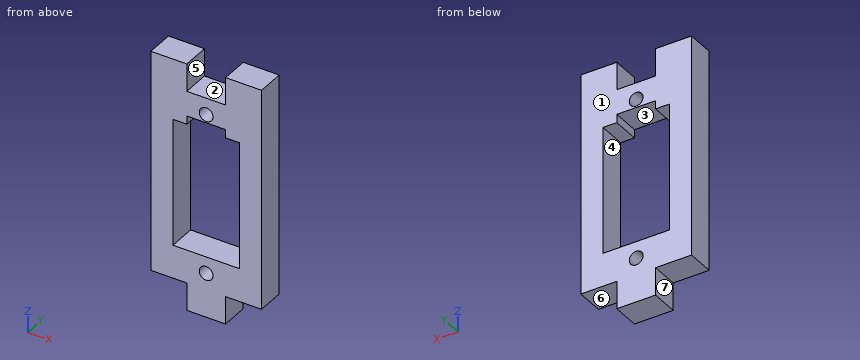
from build123d import *

# Parameters (mm, degrees)
BOSS_EXTRUDE1_DEPTH = 5
SKETCH2_R           = 1.25
CUT_EXTRUDE1_DEPTH  = 5


with BuildPart() as part:
    # Sketch1 → Boss-Extrude1 (new body)
    with BuildSketch(Plane(origin=(0, 0, 0), x_dir=(1, 0, 0), z_dir=(0, 1, 0))):
        Polygon((-10, 20), (-10, -20), (-3.5, -20), (-3.5, -15), (3.5, -15), (3.5, -20), (10, -20), (10, 20), (3.5, 20), (3.5, 25), (-3.5, 25), (-3.5, 20), align=None)
    extrude(amount=BOSS_EXTRUDE1_DEPTH)

    # Sketch2 → Cut-Extrude1 (cut)
    with BuildSketch(Plane(origin=(0, 5, 0), x_dir=(1, 0, 0), z_dir=(0, 1, 0))):
        with Locations(Location((0, 17, 0), (0, 0, 270))):
            Circle(SKETCH2_R)
        with Locations(Location((0, -12, 0), (0, 0, 270))):
            Circle(SKETCH2_R)
        Polygon((-6, 14), (6, 14), (6, -9), (3.5, -9), (3.5, -10.5), (-3.5, -10.5), (-3.5, -9), (-6, -9), align=None)
    extrude(amount=-CUT_EXTRUDE1_DEPTH, mode=Mode.SUBTRACT)


solid = part.part
The listing builds one solid part. Answer for the finished solid, in the listing's coordinates (mm). Face numbers are marked on the shaded views. A direction names the side the tool comes from. Round coordinates to 2 decimals unless told otherwise and drop trailing zeros. Write each loop counter-clockwise with the first axis right and the second up, starting at its lowest first coordinate (ties: lowest second). Pieces come first, ordered by that corner, then holes. Notation, with made-up numbers: (58, 38) - (69, 38) arc R30 ccw to (69, 76) - close; hole circle Ø9 at (-39, -17.75). An arc over 180 degrees is marked (long way). Use one line per item in the form item = value. Start each with the question number.
Item 1: A tool of negligible diameter and unlimited length cuts with its end or side. For the marked faces 4, 5, 6 and 7, from which of +Z, -Z, +X, -X, +Y, -Y can it reach the whole face along a straight path? Write none if from no direction.
Item 2: Find the intervals of material crossed by line 1 (Z direction, x = 2.25, y = 3.1); line 2 (X direction, y = 0.35, z = -9); line 3 (Z direction, x = 4.75, y = 0.55), in increasing order. Write a range as [from, to].
Item 3: A cutting plane is placed at D-D (x = 4.75). Write down the section's boundary in (y, z).
Item 4: A cutting plane is placed at A-A (x = 0). Write down the section's boundary in (y, z).
Item 5: Flat-ended cylindrical pins translate along their axes: pin 1 Ø1.5 at (x, y) = (-7, 2) entering from -Z; pin 2 Ø2.5 at (y, z) = (2.5, -22) entering from +X. Find the tip coordinate at first contact, or state that the pin passes through.
Item 6: Determine the mould class of the marked faces 1, 2 and 3 for opening direction Z: +Z half, -Z half, draft (parallel to the pull), parting line (faces both ways), or undercut.
Item 7: A cutting plane is placed at B-B (z = -17). Write down the section's boundary in (x, y), plus the area to 3 significant figures.
Item 8: A cutting plane is placed at C-C (y = 1.1). Write down the section's boundary in (x, z), plus the area to 3 significant figures.
The answers:
q1.face_4 = +Y, -Y
q1.face_5 = +Z, +Y, -Y
q1.face_6 = -Z, +X, +Y, -Y
q1.face_7 = -Z, -X, +Y, -Y
q2.line_1 = [-25, -14], [10.5, 15]
q2.line_2 = [-10, -6], [6, 10]
q2.line_3 = [-20, -14], [9, 20]
q3.outline = (0, -20) - (5, -20) - (5, -14) - (0, -14) - close; (0, 9) - (5, 9) - (5, 20) - (0, 20) - close
q4.outline = (0, -25) - (5, -25) - (5, -18.25) - (0, -18.25) - close; (0, -15.75) - (5, -15.75) - (5, -14) - (0, -14) - close; (0, 10.5) - (5, 10.5) - (5, 10.75) - (0, 10.75) - close; (0, 13.25) - (5, 13.25) - (5, 15) - (0, 15) - close
q5.pin_1 = -20
q5.pin_2 = 3.5
q6.face_1 = draft
q6.face_2 = +Z half
q6.face_3 = undercut
q7.outline = (-10, 0) - (-1.25, 0) - (-1.25, 5) - (-10, 5) - close; (1.25, 0) - (10, 0) - (10, 5) - (1.25, 5) - close
q7.area = 87.5 mm^2
q8.outline = (-10, -20) - (-3.5, -20) - (-3.5, -25) - (3.5, -25) - (3.5, -20) - (10, -20) - (10, 20) - (3.5, 20) - (3.5, 15) - (-3.5, 15) - (-3.5, 20) - (-10, 20) - close; hole (-6, -14) - (6, -14) - (6, 9) - (3.5, 9) - (3.5, 10.5) - (-3.5, 10.5) - (-3.5, 9) - (-6, 9) - close; hole circle Ø2.5 at (0, -17); hole circle Ø2.5 at (0, 12)
q8.area = 504 mm^2
